```python
from build123d import *

# Parameters (mm, degrees)
EXTRUDE_1_DEPTH          = 4
SKETCH_2_R               = 1.25
SKETCH_2_R_2             = 1.5
SKETCH_2_W               = 22.5
SKETCH_2_H               = 12.2
CUT_EXTRUDE_1_DEPTH      = 5
SKETCH_3_W               = 7
SKETCH_3_H               = 13
EXTRUDE_2_DEPTH          = 13
SKETCH_4_R               = 2.15
CUT_EXTRUDE_2_DEPTH      = 1
CUT_EXTRUDE_2_DEPTH_BACK = 31
FILLET_3_R               = 5
SKETCH_5_R               = 3.5
CUT_EXTRUDE_3_DEPTH      = 2
SKETCH_6_W               = 7
SKETCH_6_H               = 3
CUT_EXTRUDE_4_DEPTH      = 13
SKETCH_7_W               = 15
SKETCH_7_H               = 17
EXTRUDE_3_DEPTH          = 4
SKETCH_8_W               = 7
SKETCH_8_H               = 10
EXTRUDE_4_DEPTH          = 13
SKETCH_9_R               = 2.4
CUT_EXTRUDE_5_DEPTH      = 48


with BuildPart() as part:
    # 草图1 → 凸台-拉伸1 (new body)
    with BuildSketch(Plane.XY):
        Polygon((-30, -15), (30, -15), (30, -2), (13.5, 15), (-13.5, 15), (-30, -2), align=None)
    extrude(amount=EXTRUDE_1_DEPTH)

    # 草图2 → 切除-拉伸1 (cut, through all)
    with BuildSketch(Plane.XY.offset(4)):
        with Locations((-13.9, 3.610655805)):
            Circle(SKETCH_2_R)
        with Locations((13.9, 3.610655805)):
            Circle(SKETCH_2_R)
        with Locations((-15, -9.553859164)):
            Circle(SKETCH_2_R_2)
        with Locations((15, -9.553859164)):
            Circle(SKETCH_2_R_2)
        with Locations((0, 3.9)):
            Rectangle(SKETCH_2_W, SKETCH_2_H)
    extrude(amount=-CUT_EXTRUDE_1_DEPTH, mode=Mode.SUBTRACT)

    # 草图3 → 凸台-拉伸2 (add)
    with BuildSketch(Plane.XY.offset(4)):
        with Locations((-26.5, -8.5)):
            Rectangle(SKETCH_3_W, SKETCH_3_H)
        with Locations((26.5, -8.5)):
            Rectangle(SKETCH_3_W, SKETCH_3_H)
    extrude(amount=EXTRUDE_2_DEPTH)

    # 草图4 → 切除-拉伸2 (cut, two sides)
    with BuildSketch(Plane(origin=(0, -15, 0), x_dir=(-1, 0, 0), z_dir=(0, -1, 0))) as cut_extrude_2_sk:
        with Locations((26, -13)):
            Circle(SKETCH_4_R)
        with Locations((-26, -13)):
            Circle(SKETCH_4_R)
    extrude(amount=CUT_EXTRUDE_2_DEPTH, mode=Mode.SUBTRACT)
    extrude(cut_extrude_2_sk.sketch, amount=-CUT_EXTRUDE_2_DEPTH_BACK, mode=Mode.SUBTRACT)

    # 圆角3
    fillet_3_edges = [part.edges().sort_by_distance(p)[0] for p in [
        (-13.5, 15, 2),
        (13.5, 15, 2),
    ]]
    fillet(fillet_3_edges, radius=FILLET_3_R)

    # 草图5 → 切除-拉伸3 (cut)
    with BuildSketch(Plane.XY.offset(4)):
        with Locations((-15, -9.553859164)):
            Circle(SKETCH_5_R)
        with Locations((15, -9.553859164)):
            Circle(SKETCH_5_R)
    extrude(amount=-CUT_EXTRUDE_3_DEPTH, mode=Mode.SUBTRACT)

    # 草图6 → 切除-拉伸4 (cut)
    with BuildSketch(Plane.XY.offset(17)):
        with Locations((-26.5, -13.5)):
            Rectangle(SKETCH_6_W, SKETCH_6_H)
        with Locations((26.5, -13.5)):
            Rectangle(SKETCH_6_W, SKETCH_6_H)
    extrude(amount=-CUT_EXTRUDE_4_DEPTH, mode=Mode.SUBTRACT)

    # 草图7 → 凸台-拉伸3 (add)
    with BuildSketch(Plane.XY.offset(4)):
        with Locations((-22.5, -23.5)):
            Rectangle(SKETCH_7_W, SKETCH_7_H)
        with Locations((22.5, -23.5)):
            Rectangle(SKETCH_7_W, SKETCH_7_H)
    extrude(amount=-EXTRUDE_3_DEPTH)

    # 草图8 → 凸台-拉伸4 (add)
    with BuildSketch(Plane.XY.offset(4)):
        with Locations((-26.5, -27)):
            Rectangle(SKETCH_8_W, SKETCH_8_H)
        with Locations((26.5, -27)):
            Rectangle(SKETCH_8_W, SKETCH_8_H)
    extrude(amount=EXTRUDE_4_DEPTH)

    # 草图9 → 切除-拉伸5 (cut, through all)
    with BuildSketch(Plane.XZ.offset(32)):
        with Locations((-26, 13)):
            Circle(SKETCH_9_R)
        with Locations((26, 13)):
            Circle(SKETCH_9_R)
    extrude(amount=-CUT_EXTRUDE_5_DEPTH, mode=Mode.SUBTRACT)


solid = part.part
```
For this review, take the finished solid that the model builds, in its own axes (mm). A direction names the side the tool comes from. Give positions to 0.01 mm unless a question says otherwise; leave off trailing zeros. Order: outer loops, then holes, each group sorted by start corner. A loop starts at its lowest first (then second) coordinate and runs counter-clockwise, first axis right, second up.
1) Take a section at D-D (y = -16). Give the boundary of the cut face in (x, z).
2) For faces 1 (the face through (-11.662, -8.503, 3.014)), 2 (the face through (0, -2.2, 2)), 3 (the face through (26, -22, 10)), list the 3-axis set-ups (+Z, -Z, +X, -X, +Y, -Y) from which the entire face can be reached by the end or side of a thin tool; tool diameter is ignored.
3) Wall thickness on line 1 (Y direction, x = -24, z = 6.25); line 2 (Y direction, x = -9, z = 1.25); line 3 (X direction, y = -26, z = 6.75): over which ranges is each line inside the solid? List them lowest first.
4) Take a section at C-C (x = 7.5). Give the boundary of the cut face in (y, z).
5) Take a section at B-B (y = -28). Give the boundary of the cut face in (x, z).
6) Insertion check: pin 1 (3.5 mm diameter, centred on x = 13.5, y = -9, fed in from +Z); pin 2 (4.5 mm diameter, centred on x = 2.5, z = 1, fed in from -Y); pin 3 (1 mm diameter, centred on x = 12.5, y = -0.5, fed in from +Z). Each pin has a flat end and moves straight along its axis. Give the tip position at first contact, or say it passes through.
7) Take a section at A-A (z = 13). State how many separate pieces and enclosed holes the cut face has, then the cut area to 3 significant figures.
8) The part is to be moulded in two halves that separate along Y. For faces 4 (the face through (24, -32, 7)), 5 (the face through (17, -10, 2)), 6 (the face through (23, -27, 10)), say which applies: released by +Y, released by -Y, zero draft, split by the parting line, or undercut.
Derived:
1. outline: (-30, 0) - (-15, 0) - (-15, 4) - (-30, 4) - close; (15, 0) - (30, 0) - (30, 4) - (15, 4) - close
2. face 1: +Z
2. face 2: +Z, -Z
2. face 3: +Z, +X, -X
3. line 1: y = -32 to -22, -12 to -2
3. line 2: y = -15 to -2.2, 10 to 15
3. line 3: x = -30 to -23, 23 to 30
4. outline: (-15, 0) - (-2.2, 0) - (-2.2, 4) - (-15, 4) - close; (10, 0) - (15, 0) - (15, 4) - (10, 4) - close
5. outline: (-30, 0) - (-15, 0) - (-15, 4) - (-23, 4) - (-23, 17) - (-30, 17) - close; (15, 0) - (30, 0) - (30, 17) - (23, 17) - (23, 4) - (15, 4) - close; hole circle Ø4.8 at (-26, 13); hole circle Ø4.8 at (26, 13)
6. pin 1: stops at z = 2
6. pin 2: stops at y = -15
6. pin 3: stops at z = 4
7. separate pieces: 8
7. enclosed holes: 0
7. area: 88.0 mm2
8. face 4: released by -Y
8. face 5: undercut
8. face 6: zero draft
